Part model, mm, in its own coordinate system. Face numbers are marked on the shaded views. A direction names the side the tool comes from. Round coordinates to 2 decimals unless told otherwise and drop trailing zeros. Write each loop counter-clockwise with the first axis right and the second up, starting at its lowest first coordinate (ties: lowest second). Pieces come first, ordered by that corner, then holes. Notation, with made-up numbers: M -40,0 L 9,0 A11 cw 9,16 Z; hole C -18.5,84.25 d11. An arc over 180 degrees is marked long. Use one line per item in the form item = value. Start each with the question number.
Item 1: Flat gauge pins, fed straight in: pin 1 Ø10 at (x, y) = (41.5, -86) entering from +Z; pin 2 Ø13 at (x, y) = (42.5, -82.5) entering from -Z; pin 3 Ø5 at (x, y) = (-14.5, -50) entering from +Z; pin 4 Ø8 at (x, y) = (2, -48.5) entering from -Z. Where does each tip first touch, or does it go through?
Item 2: Probe L1, parallel to Z at x = 1, y = -51; L2, parallel to X at y = -30, z = 2; L3, parallel to Z at x = 53, y = -66.5. List the from-to ranges inside material, lowest first.
Item 3: Cut at B-B, the plane y = -78. Give the cut face in (x, z), then the cut area to 3 significant figures.
Item 4: Cut at A-A, the plane z = 3. Give the cut face in (x, y).
Item 5: Cut at D-D, the plane x = -32. Give the cut face in (y, z).
Item 6: Which spindle directions (+Z, -Z, +X, -X, +Y, -Y) get a long thin tool onto all of the face, cutting with end or side? Do the marked faces 1, 2, 3, 4 and 5. Say none if no direction does.
Item 7: Cut at C-C, the plane x = 3.5. Give the cut face in (y, z), then the cut area to 3 significant figures.
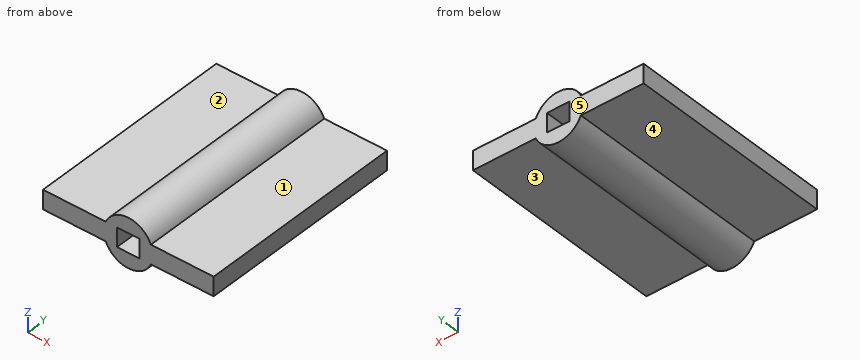
from build123d import *

# Parameters (mm, degrees)
F0_R     = 17.1435260445
F1_DEPTH = 145.1113671064
F2_W     = 15.8428698778
F2_H     = 13.308968395
F3_DEPTH = 239.869505167
F4_DEPTH = 51.8945604563
F5_DEPTH = 51.8922


with BuildPart() as f1:
    # F0 (on Front) → F1 (new body)
    with BuildSketch(Plane.XZ):
        Circle(F0_R)
    extrude(amount=F1_DEPTH)

    # F2 (on Front) → F3 (cut)
    with BuildSketch(Plane.XZ):
        Rectangle(F2_W, F2_H)
    extrude(amount=F3_DEPTH, mode=Mode.SUBTRACT)

    # F4 (add): a face of the model
    f4_faces = [f1.faces().sort_by_distance(p)[0] for p in [
        (-7.9214349389, -72.5556835532, 0),
    ]]
    extrude(f4_faces, amount=-F4_DEPTH)

    # F5 (add): a face of the model
    f5_faces = [f1.faces().sort_by_distance(p)[0] for p in [
        (7.9214349389, -72.5556835532, 0),
    ]]
    extrude(f5_faces, amount=-F5_DEPTH)


solid = f1.part
Model answer:
q1.pin_1 = 6.65
q1.pin_2 = -6.65
q1.pin_3 = 12.24
q1.pin_4 = -17.14
q2.L1 = -17.11 to -6.65, 6.65 to 17.11
q2.L2 = -59.82 to -7.92, 7.92 to 59.81
q2.L3 = -6.65 to 6.65
q3.outline = M -59.82,-6.65 L -15.8,-6.65 A17.14 ccw 15.8,-6.65 L 59.81,-6.65 L 59.81,6.65 L 15.8,6.65 A17.14 ccw -15.8,6.65 L -59.82,6.65 Z; hole M -7.92,-6.65 L 7.92,-6.65 L 7.92,6.65 L -7.92,6.65 Z
q3.area = 1,860 mm²
q4.outline = M -59.82,-145.11 L -7.92,-145.11 L -7.92,0 L -59.82,0 Z; M 7.92,-145.11 L 59.81,-145.11 L 59.81,0 L 7.92,0 Z
q5.outline = M -145.11,-6.65 L 0,-6.65 L 0,6.65 L -145.11,6.65 Z
q6.face_1 = +Z, +X, +Y, -Y
q6.face_2 = +Z, -X, +Y, -Y
q6.face_3 = -Z, +X, +Y, -Y
q6.face_4 = -Z, -X, +Y, -Y
q6.face_5 = +Z, -Z, +X, -X, +Y
q7.outline = M -145.11,-16.78 L 0,-16.78 L 0,-6.65 L -145.11,-6.65 Z; M -145.11,6.65 L 0,6.65 L 0,16.78 L -145.11,16.78 Z
q7.area = 2,940 mm²
